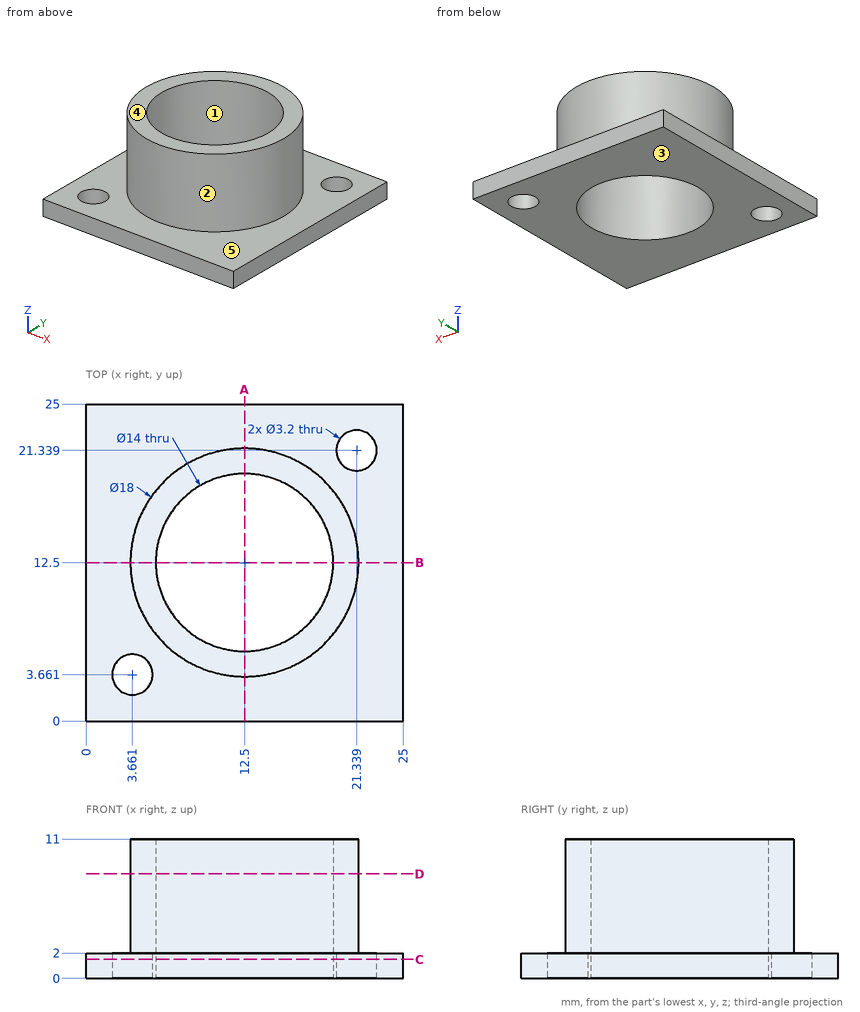
Could you check a few things on this drawing? It's one solid part, dimensions in mm from its lowest x, y, z. A direction names the side the tool comes from. Round coordinates to 2 decimals unless told otherwise and drop trailing zeros. Order: outer loops, then holes, each group sorted by start corner. A loop starts at its lowest first (then second) coordinate and runs counter-clockwise, first axis right, second up. Notation, with made-up numbers: M 87,-21 L 108,-21 A16 ccw 108,-6 Z; hole C -31.75,-15 d2. An arc over 180 degrees is marked long. One line per item, written item: value.
(1) Imagine slicing it at C-C (z = 1.5). Write out the boundary of the cut face in (x, y), and give its area (3 significant figures).
Ans:
outline: M 0,0 L 25,0 L 25,25 L 0,25 Z; hole C 3.66,3.66 d3.2; hole C 12.5,12.5 d14; hole C 21.34,21.34 d3.2
area: 455 mm^2
(2) Imagine slicing it at A-A (x = 12.5). Write out the boundary of the cut face in (y, z).
Ans:
outline: M 0,0 L 5.5,0 L 5.5,11 L 3.5,11 L 3.5,2 L 0,2 Z; M 19.5,0 L 25,0 L 25,2 L 21.5,2 L 21.5,11 L 19.5,11 Z
(3) Imagine slicing it at D-D (z = 8.25). Write out the boundary of the cut face in (x, y).
Ans:
outline: C 12.5,12.5 d18; hole C 12.5,12.5 d14
(4) Which directions (+Z, -Z, +X, -X, +Y, -Y) give clear straight access to the entire face, cutting with the end or side of a thin tool? Please do the marked faces 4 and 5.
Ans:
face 4: +Z, +X, -X, +Y, -Y
face 5: +Z
(5) I need wall thicknesses on line 1 along Z through (x, y) = (15, 2); line 2 along Y through (x, z) = (12.5, 7.25); line 3 along Y through (x, z) = (18.25, 10). Which ranges of each line are inside material? Lowest first, please. Write a range as from..to.
Ans:
line 1: z = 0..2
line 2: y = 3.5..5.5, 19.5..21.5
line 3: y = 5.58..8.51, 16.49..19.42
(6) I'm going to push flat-ended pins straight in: P1, Ø3, axis at y = 15.5, z = 6.5, coming from the -X side; P2, Ø1.9, axis at x = 3.66, y = 3.66, coming from the -Z side; P3, Ø1.5, axis at y = 21.5, z = 3.5, coming from the -X side; P4, Ø3, axis at x = 3, z = 4, coming from the -Y side. Where does each tip first touch, or does it pass through?
Ans:
P1: stops at x = 3.63
P2: passes through
P3: stops at x = 8.9
P4: stops at y = 8.38
(7) If we mould it in two halves opening along Y, with no side actions, what happens to the marked faces 1, 2 and 3? For each: released by +Y, released by -Y, zero draft, split by the parting line, or undercut.
Ans:
face 1: undercut
face 2: split by the parting line
face 3: zero draft
